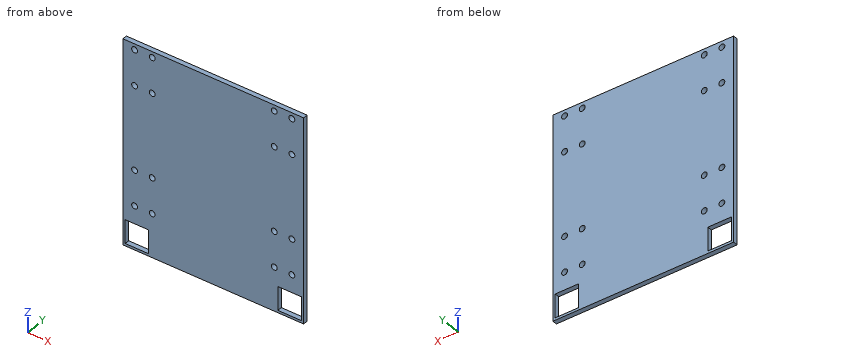
```python
from build123d import *

# Parameters (mm, degrees)
SKETCH1_W           = 154
SKETCH1_H           = 173
BOSS_EXTRUDE1_DEPTH = 4
SKETCH2_R           = 2.5
SKETCH2_W           = 20
SKETCH2_H           = 20
CUT_EXTRUDE1_DEPTH  = 4


with BuildPart() as part:
    # Sketch1 → Boss-Extrude1 (new body)
    with BuildSketch(Plane(origin=(0, 0, 0), x_dir=(1, 0, 0), z_dir=(0, 1, 0))):
        with Locations((-77, -86.5)):
            Rectangle(SKETCH1_W, SKETCH1_H)
    extrude(amount=BOSS_EXTRUDE1_DEPTH)

    # Sketch2 → Cut-Extrude1 (cut)
    with BuildSketch(Plane(origin=(0, 4, 0), x_dir=(1, 0, 0), z_dir=(0, 1, 0))):
        with Locations(Location((-144, -37, 0), (0, 0, 270))):
            Circle(SKETCH2_R)
        with Locations(Location((-129, -37, 0), (0, 0, 270))):
            Circle(SKETCH2_R)
        with Locations(Location((-144, -67, 0), (0, 0, 270))):
            Circle(SKETCH2_R)
        with Locations(Location((-129, -67, 0), (0, 0, 270))):
            Circle(SKETCH2_R)
        with Locations(Location((-25, -67, 0), (0, 0, 90))):
            Circle(SKETCH2_R)
        with Locations(Location((-10, -67, 0), (0, 0, 90))):
            Circle(SKETCH2_R)
        with Locations(Location((-25, -37, 0), (0, 0, 90))):
            Circle(SKETCH2_R)
        with Locations(Location((-10, -37, 0), (0, 0, 90))):
            Circle(SKETCH2_R)
        with Locations(Location((-10, -168, 0), (0, 0, 270))):
            Circle(SKETCH2_R)
        with Locations(Location((-25, -168, 0), (0, 0, 270))):
            Circle(SKETCH2_R)
        with Locations(Location((-10, -138, 0), (0, 0, 270))):
            Circle(SKETCH2_R)
        with Locations(Location((-25, -138, 0), (0, 0, 270))):
            Circle(SKETCH2_R)
        with Locations(Location((-129, -138, 0), (0, 0, 90))):
            Circle(SKETCH2_R)
        with Locations(Location((-144, -138, 0), (0, 0, 90))):
            Circle(SKETCH2_R)
        with Locations(Location((-129, -168, 0), (0, 0, 90))):
            Circle(SKETCH2_R)
        with Locations(Location((-144, -168, 0), (0, 0, 90))):
            Circle(SKETCH2_R)
        with Locations((-142, -12)):
            Rectangle(SKETCH2_W, SKETCH2_H)
        with Locations((-12, -12)):
            Rectangle(SKETCH2_W, SKETCH2_H)
    extrude(amount=-CUT_EXTRUDE1_DEPTH, mode=Mode.SUBTRACT)


solid = part.part
```
Work out the finished part from the listing and answer in its coordinate system (mm). Give positions to 0.01 mm unless a question says otherwise; leave off trailing zeros. Write each loop counter-clockwise with the first axis right and the second up, starting at its lowest first coordinate (ties: lowest second). Pieces come first, ordered by that corner, then holes. Notation, with made-up numbers: (-6.75, -33) - (10.25, -33) arc R28 ccw to (10.25, -1) - close; hole circle Ø3 at (52.25, 40). An arc over 180 degrees is marked (long way). Use one line per item in the form item = value.
1. This flat-tipped pin is pushed along its axis until it touches: pin 1 Ø3 at (x, z) = (-25, 67) entering from -Y. Where does it stop, or does it pass through?
Filled in:
pin_1 = through
2. A cutting plane is placed at D-D (x = -134). Write down the section's boundary in (y, z).
Filled in:
outline = (0, 0) - (4, 0) - (4, 2) - (0, 2) - close; (0, 22) - (4, 22) - (4, 173) - (0, 173) - close
3. A cutting plane is placed at B-B (z = 37). Write down the section's boundary in (x, y).
Filled in:
outline = (-154, 0) - (-146.5, 0) - (-146.5, 4) - (-154, 4) - close; (-141.5, 0) - (-131.5, 0) - (-131.5, 4) - (-141.5, 4) - close; (-126.5, 0) - (-27.5, 0) - (-27.5, 4) - (-126.5, 4) - close; (-22.5, 0) - (-12.5, 0) - (-12.5, 4) - (-22.5, 4) - close; (-7.5, 0) - (0, 0) - (0, 4) - (-7.5, 4) - close
4. Consider L1, parallel to X at y = 2.45, z = 37; L2, parallel to Z at x = -144, y = 1.2; L3, parallel to Z at x = -129, y = 1.45. Determine where each line is inside the solid, lowest interval first.
Filled in:
L1 = -154 to -146.5, -141.5 to -131.5, -126.5 to -27.5, -22.5 to -12.5, -7.5 to 0
L2 = 0 to 2, 22 to 34.5, 39.5 to 64.5, 69.5 to 135.5, 140.5 to 165.5, 170.5 to 173
L3 = 0 to 34.5, 39.5 to 64.5, 69.5 to 135.5, 140.5 to 165.5, 170.5 to 173
5. A cutting plane is placed at A-A (x = -10). Write down the section's boundary in (y, z), and give its area (3 significant figures).
Filled in:
outline = (0, 0) - (4, 0) - (4, 2) - (0, 2) - close; (0, 22) - (4, 22) - (4, 34.5) - (0, 34.5) - close; (0, 39.5) - (4, 39.5) - (4, 64.5) - (0, 64.5) - close; (0, 69.5) - (4, 69.5) - (4, 135.5) - (0, 135.5) - close; (0, 140.5) - (4, 140.5) - (4, 165.5) - (0, 165.5) - close; (0, 170.5) - (4, 170.5) - (4, 173) - (0, 173) - close
area = 532 mm^2
6. A cutting plane is placed at C-C (y = 2.1). State how many separate pieces and enclosed holes the cut face has, and give its area (3 significant figures).
Filled in:
separate_pieces = 1
enclosed_holes = 18
area = 25,500 mm^2
